Verification items for the finished model (mm, model axes). Round coordinates to 2 decimals unless told otherwise and drop trailing zeros. Order: outer loops, then holes, each group sorted by start corner. A loop starts at its lowest first (then second) coordinate and runs counter-clockwise, first axis right, second up. Notation, with made-up numbers: (-11.5, 10.25) -> (11.5, 10.25) arc R16 ccw to (11.5, 32.25) -> close; hole circle Ø9 at (30.5, 71). An arc over 180 degrees is marked (long way). Put each result on its own line as item: value.
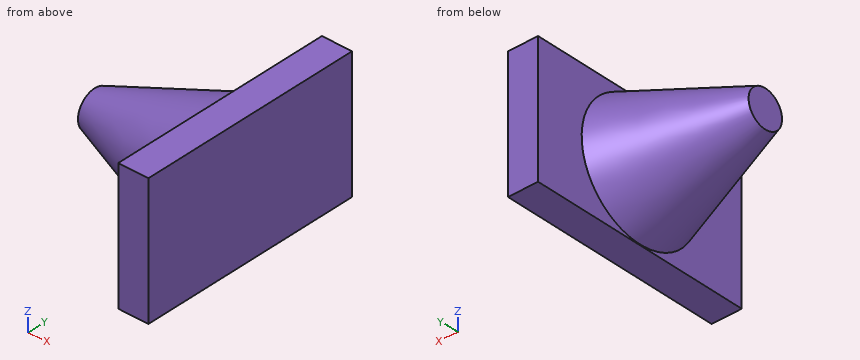
from build123d import *

# Parameters (mm, degrees)
F2_T     = -3.3
F3_W     = 45
F3_H     = 26.067962
F4_DEPTH = 6


with BuildPart() as f1:
    # F0 (on Front) → F1 (revolve)
    with BuildSketch(Plane.XZ):
        Polygon((-21.407768, 3.695389), (-21.407768, 0), (3.567961, 0), (3.567961, 12.870146), align=None)
    revolve(axis=Axis((-8.919903, 0, 0), (-1, 0, 0)))

    # F2
    f2_openings = [f1.faces().sort_by_distance(p)[0] for p in [
        (3.567961, 0, 0),
    ]]
    offset(amount=F2_T, openings=f2_openings)

    # F3 (on face) → F4 (join)
    with BuildSketch(Plane.YZ.offset(3.567961)):
        Rectangle(F3_W, F3_H)
    extrude(amount=F4_DEPTH)


solid = f1.part
Item 1: Section check B-B on z = 0. Record the boundary of the cut face in (x, y).
Check sheet entries:
outline: (-21.41, -3.7) -> (3.57, -12.87) -> (3.57, -22.5) -> (9.57, -22.5) -> (9.57, 22.5) -> (3.57, 22.5) -> (3.57, 12.87) -> (-21.41, 3.7) -> close; hole (-18.11, -1.39) -> (3.57, -9.35) -> (3.57, 9.35) -> (-18.11, 1.39) -> close
Item 2: Material ranges on L1, parallel to X at y = -19.5, z = -5.5; L2, parallel to Y at x = 1, z = 3.75; L3, parallel to X at y = -5.5, z = -2.75, recorded low to high. Write a range as [from, to].
Check sheet entries:
L1: x = [3.57, 9.57]
L2: y = [-11.32, -7.53], [7.53, 11.32]
L3: x = [-14.73, -5.16], [3.57, 9.57]
Item 3: Section check C-C on x = -16. Record the boundary of the cut face in (y, z), then the cut area to 3 significant figures.
Check sheet entries:
outline: circle Ø11.36 at (0, 0); hole circle Ø4.33 at (0, 0)
area: 86.7 mm^2
Item 4: Section check D-D on y = 14. Record the boundary of the cut face in (x, z).
Check sheet entries:
outline: (3.57, -13.03) -> (9.57, -13.03) -> (9.57, 13.03) -> (3.57, 13.03) -> close
Item 5: Section check A-A on y = 0. Record the boundary of the cut face in (x, z), then the cut area to 3 significant figures.
Check sheet entries:
outline: (-21.41, -3.7) -> (3.57, -12.87) -> (3.57, -13.03) -> (9.57, -13.03) -> (9.57, 13.03) -> (3.57, 13.03) -> (3.57, 12.87) -> (-21.41, 3.7) -> close; hole (-18.11, -1.39) -> (3.57, -9.35) -> (3.57, 9.35) -> (-18.11, 1.39) -> close
area: 337 mm^2
Item 6: Gauge pin test, flat ends, axial feed: pin 1 Ø4 at (x, z) = (-8.5, 2) entering from -Y; pin 2 Ø2 at (x, z) = (-4.5, 9) entering from -Y; pin 3 Ø1.5 at (x, y) = (-10.5, -6.5) entering from +Z. Record the tip position at first contact, or that the pin passes through.
Check sheet entries:
pin 1: stops at y = -9.03
pin 2: stops at y = -5.98
pin 3: stops at z = 5.22
